from build123d import *

# Parameters (mm, degrees)
SKICA1_R                 = 55
P_IDAT_VYSUNUT_M1_DEPTH  = 93
SKICA3_R                 = 52.5
ODEBRAT_VYSUNUT_M1_DEPTH = 90
SKICA5_R                 = 2.5
ODEBRAT_VYSUNUT_M5_DEPTH = 90


with BuildPart() as part:
    # Skica1 → Přidat vysunutím1 (new body)
    with BuildSketch(Plane.XY):
        with Locations(Location((0, 0, 0), (0, 0, 180))):
            Circle(SKICA1_R)
    extrude(amount=P_IDAT_VYSUNUT_M1_DEPTH)

    # Skica3 → Odebrat vysunutím1 (cut)
    with BuildSketch(Plane.XY.offset(93)):
        Circle(SKICA3_R)
    extrude(amount=-ODEBRAT_VYSUNUT_M1_DEPTH, mode=Mode.SUBTRACT)

    # Skica5 → Odebrat vysunutím5 (cut)
    with BuildSketch(Plane(origin=(0, 0, 0), x_dir=(-1, 0, 0), z_dir=(0, 0, -1))):
        Circle(SKICA5_R)
        with BuildLine():
            Line((0, -4.754963748), (0, -52.754963748))
            ThreePointArc((0, -52.754963748), (37.280920542, -37.291104979), (52.72020336, 0))
            Line((52.72020336, 0), (4.72020336, 0))
            Line((4.72020336, 0), (0, -4.754963748))
        make_face()
    extrude(amount=-ODEBRAT_VYSUNUT_M5_DEPTH, mode=Mode.SUBTRACT)


solid = part.part
Geometry: final body of the model. Coordinates: model frame, mm. A direction names the side the tool comes from. Coordinates: 2 decimals unless noted, no trailing zeros. Write each loop counter-clockwise with the first axis right and the second up, starting at its lowest first coordinate (ties: lowest second). Pieces come first, ordered by that corner, then holes. Notation, with made-up numbers: (60.25, -26.5) - (86.25, -26.5) arc R23 cw to (86.25, 10.5) - close; hole circle Ø2 at (20.5, -39.75). An arc over 180 degrees is marked (long way). Return JSON: item names as keys, results as strings.
Item 1: Pin query (flat end, axial travel): pin 1 Ø4 at (x, y) = (15.5, 33.5) entering from -Z; pin 2 Ø2 at (y, z) = (-15, 21.5) entering from -X; pin 3 Ø8 at (x, z) = (-7.5, 43.5) entering from -Y; pin 4 Ø10 at (y, z) = (-30, 42.5) entering from +X. Return the tip coordinate at first contact, or that it passes through.
Completed:
{"pin 1": "stops at z = 0", "pin 2": "stops at x = -53.19", "pin 3": "stops at y = -54.89", "pin 4": "stops at x = 48.99"}
Item 2: Line query: L1, parallel to Z at x = 13, y = 25; L2, parallel to Y at x = -5, z = 26; L3, parallel to X at y = -34, z = 17.5. Output: solid intervals per line, ascending.
Completed:
{"L1": "z = 0 to 3", "L2": "y = -54.77 to -52.51, 52.26 to 54.77", "L3": "x = -43.23 to -40.3, 40 to 43.23"}
Item 3: Section query B-B (x = -20.5). Output: boundary loops of the cut face in (y, z).
Completed:
{"outline": "(-51.04, 0) - (-48.59, 0) - (-48.59, 90) - (-48.33, 90) - (-48.33, 93) - (-51.04, 93) - close; (0, 0) - (51.04, 0) - (51.04, 93) - (48.33, 93) - (48.33, 3) - (0, 3) - close"}
Item 4: Reachability of faces 1 (the face through (-20, 49, 93)), 2 (the face through (13, 11, 0)), 3 (the face through (-36.87, -37.7, 44.37)), 4 (the face through (11, 12, 3)), 5 (the face through (-2.393, -2.344, 1.479)) from +Z, -Z, +X, -X, +Y, -Y: full face, straight path, thin tool, end or side. Return the list, or none.
Completed:
{"face 1": "+Z, +X, -X, +Y, -Y", "face 2": "-Z, +X, -X, +Y, -Y", "face 3": "-Z", "face 4": "+Z", "face 5": "+Z, -Z"}
Item 5: Section query C-C (z = 58). Output: boundary loops of the cut face in (x, y).
Completed:
{"outline": "circle Ø110 at (0, 0); hole (-52.72, 0) arc R52.75 ccw to (0, -52.75) - (0, -52.5) arc R52.5 ccw (long way) to (-52.5, 0) - close"}
Item 6: Section query D-D (x = 37). Output: boundary loops of the cut face in (y, z), and give its area (3 significant figures).
Completed:
{"outline": "(-40.69, 0) - (40.69, 0) - (40.69, 93) - (37.25, 93) - (37.25, 3) - (-37.25, 3) - (-37.25, 93) - (-40.69, 93) - close", "area": "865 mm2"}
Item 7: Section query A-A (y = -10.5). Output: boundary loops of the cut face in (x, z).
Completed:
{"outline": "(-53.99, 0) - (-51.66, 0) - (-51.66, 90) - (-51.44, 90) - (-51.44, 93) - (-53.99, 93) - close; (0, 0) - (53.99, 0) - (53.99, 93) - (51.44, 93) - (51.44, 3) - (0, 3) - close"}
